```python
from build123d import *

# Parameters (mm, degrees)
SKETCH1_W                     = 347.98
SKETCH1_H                     = 129.54
BOSS_EXTRUDE1_DEPTH           = 6.35
TAP_DRILL_FOR_6_32_TAP4_D     = 2.7051
TAP_DRILL_FOR_6_32_TAP4_DEPTH = 17.78
TAP_DRILL_FOR_6_32_TAP4_TIP   = 0.81269403
TAP_DRILL_FOR_6_32_TAP1_D     = 2.7051
TAP_DRILL_FOR_6_32_TAP1_DEPTH = 17.78
TAP_DRILL_FOR_6_32_TAP1_TIP   = 0.81269403
TAP_DRILL_FOR_6_32_TAP2_D     = 2.7051
TAP_DRILL_FOR_6_32_TAP2_DEPTH = 17.78
TAP_DRILL_FOR_6_32_TAP2_TIP   = 0.81269403
SKETCH10_R                    = 0.889
SKETCH10_R_2                  = 1.5875
SKETCH10_R_3                  = 2.55
CUT_EXTRUDE1_DEPTH            = 7.35
SKETCH15_R                    = 6.35
CUT_EXTRUDE2_DEPTH            = 4.7625
TAP_DRILL_FOR_6_32_TAP5_D     = 2.7051
TAP_DRILL_FOR_6_32_TAP5_DEPTH = 17.78
TAP_DRILL_FOR_6_32_TAP5_TIP   = 0.81269403


with BuildPart() as part:
    # Sketch1 → Boss-Extrude1 (new body)
    with BuildSketch(Plane.XY):
        with Locations((173.99, 64.77)):
            Rectangle(SKETCH1_W, SKETCH1_H)
    extrude(amount=BOSS_EXTRUDE1_DEPTH)

    # Tap Drill for #6-32 Tap4
    with Locations(Plane(origin=(0, 13.303154199, -243.112488364), x_dir=(0, 0, 1), z_dir=(-1, 0, 0))):
        with Locations((-105.502511636, 81.946845801), (-105.502511636, 56.546845801), (-105.502511636, 31.146845801), (246.287488364, 83.216845801), (246.287488364, 51.466845801), (246.287488364, 19.716845801)):
            Hole(TAP_DRILL_FOR_6_32_TAP4_D / 2, depth=TAP_DRILL_FOR_6_32_TAP4_DEPTH)
            with Locations((0, 0, -(TAP_DRILL_FOR_6_32_TAP4_DEPTH + TAP_DRILL_FOR_6_32_TAP4_TIP / 2))):  # 118° drill point
                Cone(0, TAP_DRILL_FOR_6_32_TAP4_D / 2, TAP_DRILL_FOR_6_32_TAP4_TIP, mode=Mode.SUBTRACT)

    # Tap Drill for #6-32 Tap1
    with Locations(Plane(origin=(-62.924888364, 129.54, 269.187551164), x_dir=(0, 0, -1), z_dir=(0, 1, 0))):
        with Locations((266.012551164, -131.377888364), (266.012551164, -201.735888364), (266.012551164, -272.093888364), (266.012551164, -342.451888364)):
            Hole(TAP_DRILL_FOR_6_32_TAP1_D / 2, depth=TAP_DRILL_FOR_6_32_TAP1_DEPTH)
            with Locations((0, 0, -(TAP_DRILL_FOR_6_32_TAP1_DEPTH + TAP_DRILL_FOR_6_32_TAP1_TIP / 2))):  # 118° drill point
                Cone(0, TAP_DRILL_FOR_6_32_TAP1_D / 2, TAP_DRILL_FOR_6_32_TAP1_TIP, mode=Mode.SUBTRACT)

    # Tap Drill for #6-32 Tap2
    with Locations(Plane(origin=(-62.924888364, 0, 269.187551164), x_dir=(0, 0, 1), z_dir=(0, -1, 0))):
        with Locations((-266.012551164, -342.451888364), (-266.012551164, -272.093888364), (-266.012551164, -201.735888364), (-266.012551164, -131.377888364)):
            Hole(TAP_DRILL_FOR_6_32_TAP2_D / 2, depth=TAP_DRILL_FOR_6_32_TAP2_DEPTH)
            with Locations((0, 0, -(TAP_DRILL_FOR_6_32_TAP2_DEPTH + TAP_DRILL_FOR_6_32_TAP2_TIP / 2))):  # 118° drill point
                Cone(0, TAP_DRILL_FOR_6_32_TAP2_D / 2, TAP_DRILL_FOR_6_32_TAP2_TIP, mode=Mode.SUBTRACT)

    # Sketch10 → Cut-Extrude1 (cut, through all)
    with BuildSketch(Plane.XY.offset(6.35)):
        with Locations((335.136, 15.9564)):
            Circle(SKETCH10_R)
        with Locations((317.136, 15.9564)):
            Circle(SKETCH10_R)
        with Locations((338.1248, 56.6293)):
            Circle(SKETCH10_R_2)
        with Locations((314.1472, 47.6377)):
            Circle(SKETCH10_R_2)
        with Locations((326.136, 32.7814)):
            Circle(SKETCH10_R_3)
        with BuildLine():
            Line((313.4995, 124.841), (338.7725, 124.841))
            ThreePointArc((338.7725, 124.841), (339.895032015, 124.376032015), (340.36, 123.2535))
            Line((340.36, 123.2535), (340.36, 70.5231))
            ThreePointArc((340.36, 70.5231), (339.895032015, 69.400567985), (338.7725, 68.9356))
            Line((338.7725, 68.9356), (313.4995, 68.9356))
            ThreePointArc((313.4995, 68.9356), (312.376967985, 69.400567985), (311.912, 70.5231))
            Line((311.912, 70.5231), (311.912, 123.2535))
            ThreePointArc((311.912, 123.2535), (312.376967985, 124.376032015), (313.4995, 124.841))
        make_face()
        with BuildLine():
            Line((331.2985, 20.7064), (320.9735, 20.7064))
            ThreePointArc((320.9735, 20.7064), (319.850967985, 20.241432015), (319.386, 19.1189))
            Line((319.386, 19.1189), (319.386, 12.7939))
            ThreePointArc((319.386, 12.7939), (319.850967985, 11.671367985), (320.9735, 11.2064))
            Line((320.9735, 11.2064), (331.2985, 11.2064))
            ThreePointArc((331.2985, 11.2064), (332.421032015, 11.671367985), (332.886, 12.7939))
            Line((332.886, 12.7939), (332.886, 19.1189))
            ThreePointArc((332.886, 19.1189), (332.421032015, 20.241432015), (331.2985, 20.7064))
        make_face()
        with BuildLine():
            Line((332.8289, 59.4106), (319.4431, 59.4106))
            ThreePointArc((319.4431, 59.4106), (318.320567985, 58.945632015), (317.8556, 57.8231))
            Line((317.8556, 57.8231), (317.8556, 46.4439))
            ThreePointArc((317.8556, 46.4439), (318.320567985, 45.321367985), (319.4431, 44.8564))
            Line((319.4431, 44.8564), (332.8289, 44.8564))
            ThreePointArc((332.8289, 44.8564), (333.951432015, 45.321367985), (334.4164, 46.4439))
            Line((334.4164, 46.4439), (334.4164, 57.8231))
            ThreePointArc((334.4164, 57.8231), (333.951432015, 58.945632015), (332.8289, 59.4106))
        make_face()
    extrude(amount=-CUT_EXTRUDE1_DEPTH, mode=Mode.SUBTRACT)

    # Sketch15 → Cut-Extrude2 (cut)
    with BuildSketch(Plane.XY.offset(6.35)):
        with Locations((326.136, 32.7814)):
            Circle(SKETCH15_R)
    extrude(amount=-CUT_EXTRUDE2_DEPTH, mode=Mode.SUBTRACT)

    # Tap Drill for #6-32 Tap5
    with Locations(Plane(origin=(347.98, 0, 0), x_dir=(0, 0, -1), z_dir=(1, 0, 0))):
        with Locations((-3.175, 64.77), (-3.175, 96.52), (-3.175, 33.02)):
            Hole(TAP_DRILL_FOR_6_32_TAP5_D / 2, depth=TAP_DRILL_FOR_6_32_TAP5_DEPTH)
            with Locations((0, 0, -(TAP_DRILL_FOR_6_32_TAP5_DEPTH + TAP_DRILL_FOR_6_32_TAP5_TIP / 2))):  # 118° drill point
                Cone(0, TAP_DRILL_FOR_6_32_TAP5_D / 2, TAP_DRILL_FOR_6_32_TAP5_TIP, mode=Mode.SUBTRACT)


solid = part.part
```
CAD build for the part. Positions are in the model's coordinates, mm. A direction names the side the tool comes from. Round coordinates to 2 decimals unless told otherwise and drop trailing zeros. Answer in a Markdown table with one row per item. Add a question column.
(1) Mould opens along X. For faces 1 (the face through (0, 64, 5)), 2 (the face through (326, 124.841, 3)), 3 (the face through (172, 0, 3)), 4 (the face through (326, 59.411, 3)) say: +X half, -X half, draft (parallel to the pull), parting line (faces both ways), or undercut.
(2) Drop flat-ended pins along their axis: pin 1 Ø1.6 at (y, z) = (33.02, 3.175) entering from +X; pin 2 Ø2.5 at (x, y) = (335.14, 15.96) entering from +Z; pin 3 Ø3 at (x, y) = (326.14, 32.78) entering from -Z. Give the stop position or say it passes through.
(3) 3-axis set-ups, long thin cutter, end or side, ignore diameter. For faces 5 (the face through (334.416, 52, 3)), 6 (the face through (172, 66, 0)), 7 (the face through (332, 30.35, 4)): which of +Z, -Z, +X, -X, +Y, -Y reach the whole face in a straight line?
(4) Probe L1, parallel to X at y = 13.5, z = 3.25; L2, parallel to X at y = 107, z = 1; L3, parallel to X at y = 52.5, z = 5. List the from-to ranges inside material, lowest first. Write a range as [from, to].
Data:
| question | item | result |
|---|---|---|
| 1 | face 1 | -X half |
| 1 | face 2 | undercut |
| 1 | face 3 | draft |
| 1 | face 4 | undercut |
| 2 | pin 1 | stops at x = 319.87 |
| 2 | pin 2 | stops at z = 6.35 |
| 2 | pin 3 | passes through |
| 3 | face 5 | +Z, -Z |
| 3 | face 6 | -Z, +X, -X, +Y, -Y |
| 3 | face 7 | +Z |
| 4 | L1 | x = [0, 67.1], [69.8, 137.46], [140.16, 207.82], [210.52, 278.18], [280.88, 319.39], [332.89, 347.98] |
| 4 | L2 | x = [0, 311.91], [340.36, 347.98] |
| 4 | L3 | x = [0, 317.86], [334.42, 347.98] |
